```python
from build123d import *

# Parameters (mm, degrees)
SKETCH_1_W          = 79
SKETCH_1_H          = 27
EXTRUDE_1_DEPTH     = 10
SKETCH_3_R          = 7.5
CUT_EXTRUDE_1_DEPTH = 43.924352063
FILLET_1_R          = 3


with BuildPart() as part:
    # 草图1 → 凸台-拉伸1 (new body)
    with BuildSketch(Plane(origin=(0, 0, 0), x_dir=(1, 0, 0), z_dir=(0, 1, 0))):
        Rectangle(SKETCH_1_W, SKETCH_1_H)
    extrude(amount=EXTRUDE_1_DEPTH)

    # 草图3 → 切除-拉伸1 (cut, through all)
    with BuildSketch(Plane(origin=(0, 10, 0), x_dir=(1, 0, 0), z_dir=(0, 1, 0))):
        with Locations(Location((-27, 0, 0), (0, 0, 270))):
            Circle(SKETCH_3_R)
        with Locations(Location((27, 0, 0), (0, 0, 270))):
            Circle(SKETCH_3_R)
    extrude(amount=-CUT_EXTRUDE_1_DEPTH, mode=Mode.SUBTRACT)

    # 圆角1
    fillet_1_edges = [part.edges().sort_by_distance(p)[0] for p in [
        (39.5, 5, 13.5),
    ]]
    fillet(fillet_1_edges, radius=FILLET_1_R)


solid = part.part
```
The listing builds one solid part. Answer for the finished solid, in the listing's coordinates (mm). Coordinates: 2 decimals unless noted, no trailing zeros. Write each loop counter-clockwise with the first axis right and the second up, starting at its lowest first coordinate (ties: lowest second). Pieces come first, ordered by that corner, then holes. Notation, with made-up numbers: (59, 39.5) - (72, 39.5) arc R11 ccw to (72, 43.5) - close; hole circle Ø3 at (40, -35). An arc over 180 degrees is marked (long way). Return JSON: item names as keys, results as strings. Group by question number.
Q1. For a pull along Z with two mould halves and no side action, classify faces 1 (the flat face through (-1, 0, 0)), 2 (the cylindrical face through (-34.32, 5.07, -1.63)), 3 (the flat face through (-2, 5, 13.5)) as +Z half, -Z half, draft (parallel to the pull), parting line (faces both ways), or undercut.
Q2. Find the intervals of material crossed by line 1 along X through (y, z) = (5.25, 0); line 2 along X through (y, z) = (7.5, 1.75); line 3 along X through (y, z) = (2.25, 11.75), in increasing order. Write a range as [from, to].
Q3. The part is cut by section C-C on y = 1. Write down the section's boundary in (x, z), and give its area (3 significant figures).
Q4. The part is cut by section B-B on x = 27. Write down the section's boundary in (y, z), and give its area (3 significant figures).
Q5. The part is cut by section A-A on z = 0. Write down the section's boundary in (x, y).
Evaluation:
{
 "1": {"face 1": "draft", "face 2": "undercut", "face 3": "+Z half"},
 "2": {"line 1": "x = [-39.5, -34.5], [-19.5, 19.5], [34.5, 39.5]", "line 2": "x = [-39.5, -34.29], [-19.71, 19.71], [34.29, 39.5]", "line 3": "x = [-39.5, 39.23]"},
 "3": {"outline": "(-39.5, -13.5) - (39.5, -13.5) - (39.5, 10.5) arc R3 ccw to (36.5, 13.5) - (-39.5, 13.5) - close; hole circle Ø15 at (-27, 0); hole circle Ø15 at (27, 0)", "area": "1,780 mm2"},
 "4": {"outline": "(0, -13.5) - (10, -13.5) - (10, -7.5) - (0, -7.5) - close; (0, 7.5) - (10, 7.5) - (10, 13.5) - (0, 13.5) - close", "area": "120 mm2"},
 "5": {"outline": "(-39.5, 0) - (-34.5, 0) - (-34.5, 10) - (-39.5, 10) - close; (-19.5, 0) - (19.5, 0) - (19.5, 10) - (-19.5, 10) - close; (34.5, 0) - (39.5, 0) - (39.5, 10) - (34.5, 10) - close"}
}
